Study the drawing (mm; zero at the part's minimum x, y, z) and answer. A direction names the side the tool comes from. Round coordinates to 2 decimals unless told otherwise and drop trailing zeros. Order: outer loops, then holes, each group sorted by start corner. A loop starts at its lowest first (then second) coordinate and runs counter-clockwise, first axis right, second up. Notation, with made-up numbers: (28, -9.75) -> (37, -9.75) arc R32 ccw to (37, 19.25) -> close; hole circle Ø11 at (65.5, 8.25). An arc over 180 degrees is marked (long way). Use one line per item in the form item = value.
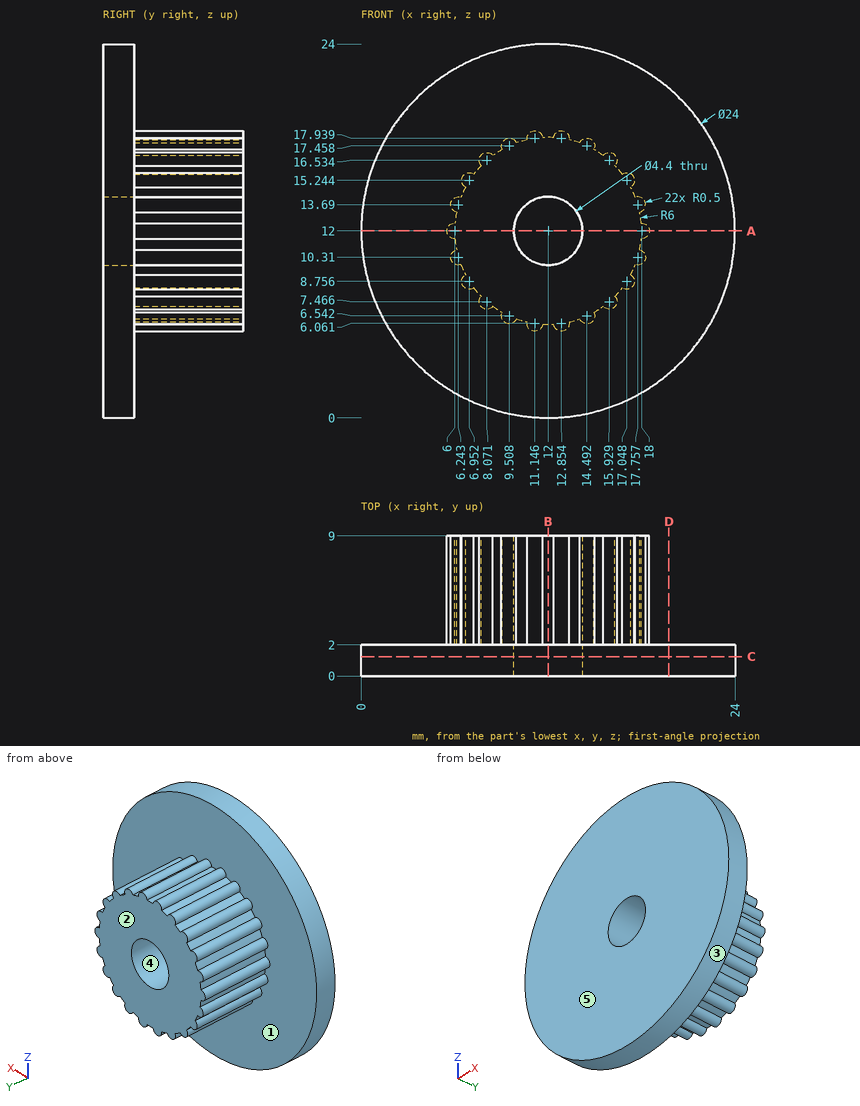
Item 1: The part is cut by section A-A, the plane z = 12. Give the vertices of the cut face in (x, y).
Findings:
outline = (0, 0) -> (9.8, 0) -> (9.8, 9) -> (5.5, 9) -> (5.5, 2) -> (0, 2) -> close; (14.2, 0) -> (24, 0) -> (24, 2) -> (18.5, 2) -> (18.5, 9) -> (14.2, 9) -> close
Item 2: For the marked faces 1 and 2, determine the directions among +Z, -Z, +X, -X, +Y, -Y from which every point of the face is accessible in a straight line to the end or side of a thin tool.
Findings:
face_1 = +Y
face_2 = +Z, -Z, +X, -X, +Y
Item 3: The part is cut by section B-B, the plane x = 12. Give the vertices of the cut face in (y, z).
Findings:
outline = (0, 0) -> (2, 0) -> (2, 6) -> (9, 6) -> (9, 9.8) -> (0, 9.8) -> close; (0, 14.2) -> (9, 14.2) -> (9, 18) -> (2, 18) -> (2, 24) -> (0, 24) -> close
Item 4: The part is cut by section D-D, the plane x = 19.75. Give the vertices of the cut face in (y, z).
Findings:
outline = (0, 2.84) -> (2, 2.84) -> (2, 21.16) -> (0, 21.16) -> close
Item 5: Flat-ended cylindrical pins translate along their axes: P1, Ø5, axis at x = 11.5, y = 6, coming from the -Z side; P2, Ø1, axis at x = 15.5, z = 19, coming from the +Y side. Find the tip coordinate at first contact, or state that the pin passes through.
Findings:
P1 = 5.56
P2 = 2
Item 6: Consider line 1 along Z through (x, y) = (12, 7.25); line 2 along X through (y, z) = (2.25, 12); line 3 along Y through (x, z) = (13.5, 18.75). Determine where each line is inside the solid, lowest interval first.
Findings:
line_1 = 6 to 9.8, 14.2 to 18
line_2 = 5.5 to 9.8, 14.2 to 18.5
line_3 = 0 to 2
Item 7: Determine the mould class of the marked faces 3, 4 and 5 for opening direction X: released by +X, released by -X, zero draft, split by the parting line, or undercut.
Findings:
face_3 = split by the parting line
face_4 = undercut
face_5 = zero draft
Item 8: The part is cut by section C-C, the plane y = 1.25. Give the vertices of the cut face in (x, z), and give its area (3 significant figures).
Findings:
outline = circle Ø24 at (12, 12); hole circle Ø4.4 at (12, 12)
area = 437 mm^2
